Answer from the drawing. Dimensions are ordinates in mm from the lowest x, y and z of the part. Coordinates: 2 decimals unless noted, no trailing zeros. Write each loop counter-clockwise with the first axis right and the second up, starting at its lowest first coordinate (ties: lowest second). Pieces come first, ordered by that corner, then holes.
(1) Given pin 1 (1.3 mm diameter, centred on y = 76, z = 6, fed in from -X), flat-ended and moving along its own axis, determine where the tip first touches the part or whether it passes through.
(2) Straight lines are drawn through the part: line 1 along Y through (x, z) = (11.5, 6.35); line 2 along X through (y, z) = (55.5, 6.75); line 3 along Y through (x, z) = (140.5, 11). For each, find the intervals that lie inside material, in ascending order.
(3) The part is cut by section B-B, the plane x = 262. Determine the outline of the cut face in (y, z), and give its area (3 significant figures).
(4) The part is cut by section C-C, the plane z = 10.5. State how many separate pieces and enclosed holes the cut face has, and give its area (3 significant figures).
(5) The part is cut by section A-A, the plane x = 209.55. Determine the outline of the cut face in (y, z).
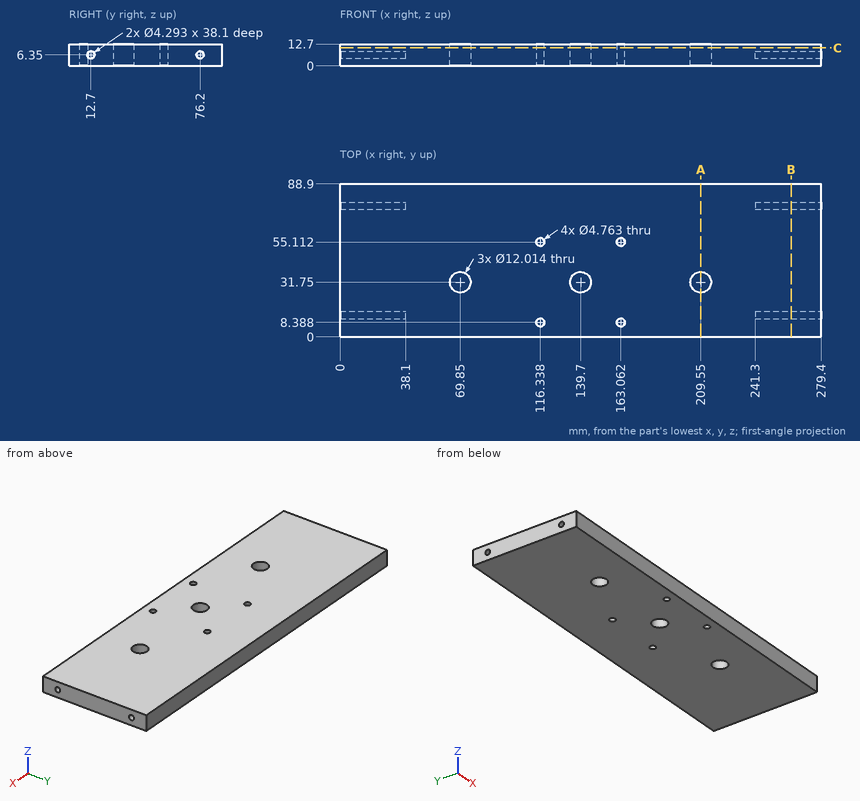
Computed:
1. pin 1: stops at x = 38.1
2. line 1: y = 0 to 10.55, 14.85 to 74.05, 78.35 to 88.9
2. line 2: x = 0 to 113.99, 118.69 to 160.71, 165.41 to 279.4
2. line 3: y = 0 to 25.8, 37.7 to 88.9
3. outline: (0, 0) - (88.9, 0) - (88.9, 12.7) - (0, 12.7) - close; hole circle Ø4.29 at (12.7, 6.35); hole circle Ø4.29 at (76.2, 6.35)
3. area: 1,100 mm2
4. separate pieces: 1
4. enclosed holes: 7
4. area: 24,400 mm2
5. outline: (0, 0) - (25.74, 0) - (25.74, 12.7) - (0, 12.7) - close; (37.76, 0) - (88.9, 0) - (88.9, 12.7) - (37.76, 12.7) - close
